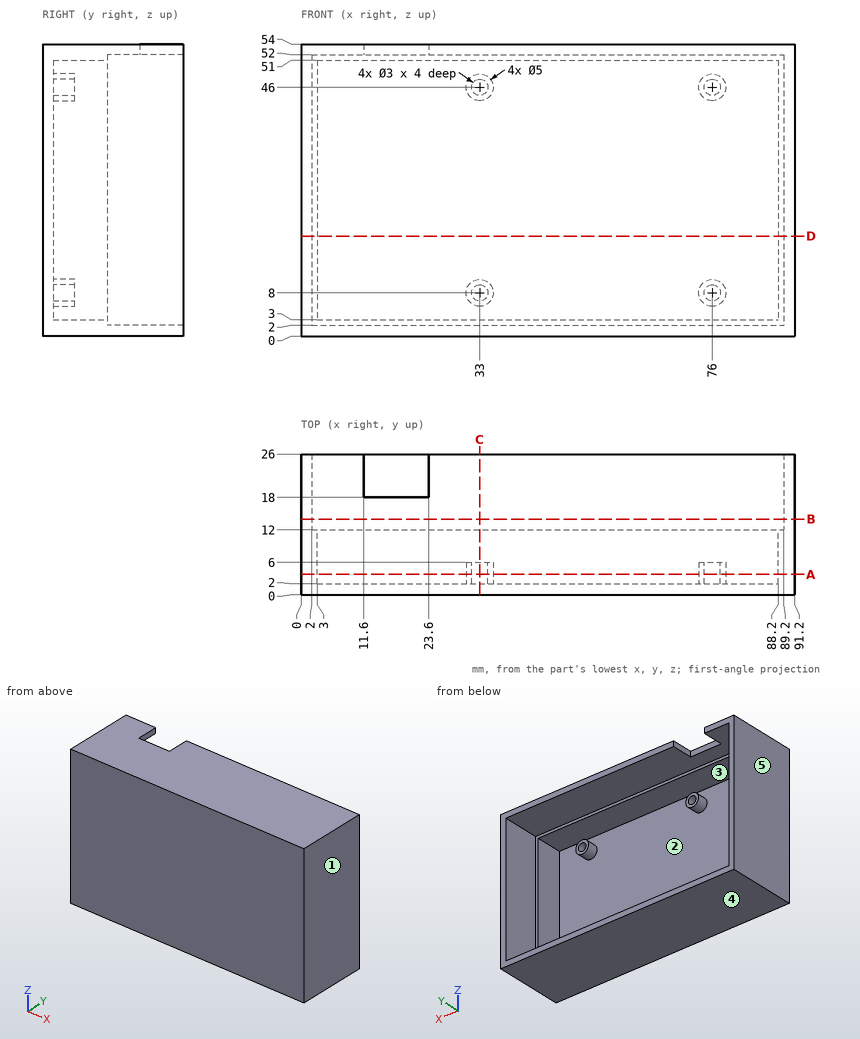
Study the drawing (mm; zero at the part's minimum x, y, z) and answer. A direction names the side the tool comes from. Give positions to 0.01 mm unless a question says otherwise; leave off trailing zeros. Write each loop counter-clockwise with the first axis right and the second up, starting at its lowest first coordinate (ties: lowest second). Pieces come first, ordered by that corner, then holes. Notation, with made-up numbers: (72.25, 60) - (101.25, 60) arc R15 cw to (101.25, 80) - close; hole circle Ø11 at (-27, -15). An arc over 180 degrees is marked (long way). Write item = value, one per line. Start each with the question number.
Item 1: Find section C-C (x = 33). Give the vertices of the cut face in (y, z), then the cut area to 3 significant figures.
Item 2: Find section A-A (y = 3.75). State how many separate pieces and enclosed holes the cut face has, then the cut area to 3 significant figures.
Item 3: Find the intervals of material crossed by probe 1 along X at (y, z) = (5.05, 8); probe 2 along Z at (x, y) = (76, 5.05); probe 3 along Z at (x, y) = (14.5, 2.75), in increasing order. Write a range as [from, to].
Item 4: Find section D-D (z = 18.5). Give the vertices of the cut face in (x, y), then the cut area to 3 significant figures.
Item 5: A tool of negligible diameter and unlimited length cuts with its end or side. For the marked faces 1 and 2, from which of +Z, -Z, +X, -X, +Y, -Y can it reach the whole face along a straight path? Write none if from no direction.
Item 6: Each of these flat-tipped pins is pushed along its axis until it touches: P1, Ø2, axis at x = 46, z = 29, coming from the +Y side; P2, Ø5.5, axis at x = 76, z = 45, coming from the +Y side; P3, Ø1.6, axis at x = 15, z = 53, coming from the +Y side. Where does it stop, or does it pass through?
Item 7: The mould has two halves that part along Z. Classify the marked faces 3, 4 and 5: +Z half, -Z half, draft (parallel to the pull), parting line (faces both ways), or undercut.
Item 8: Find section B-B (y = 14). Give the vertices of the cut face in (x, z), then the cut area to 3 significant figures.
Response:
q1.outline = (0, 0) - (26, 0) - (26, 2) - (12, 2) - (12, 3) - (2, 3) - (2, 5.5) - (6, 5.5) - (6, 6.5) - (2, 6.5) - (2, 9.5) - (6, 9.5) - (6, 10.5) - (2, 10.5) - (2, 43.5) - (6, 43.5) - (6, 44.5) - (2, 44.5) - (2, 47.5) - (6, 47.5) - (6, 48.5) - (2, 48.5) - (2, 51) - (12, 51) - (12, 52) - (26, 52) - (26, 54) - (0, 54) - close
q1.area = 240 mm²
q2.separate_pieces = 5
q2.enclosed_holes = 5
q2.area = 885 mm²
q3.probe_1 = [0, 3], [30.5, 31.5], [34.5, 35.5], [73.5, 74.5], [77.5, 78.5], [88.2, 91.2]
q3.probe_2 = [0, 3], [5.5, 6.5], [9.5, 10.5], [43.5, 44.5], [47.5, 48.5], [51, 54]
q3.probe_3 = [0, 3], [51, 54]
q4.outline = (0, 0) - (91.2, 0) - (91.2, 26) - (89.2, 26) - (89.2, 12) - (88.2, 12) - (88.2, 2) - (3, 2) - (3, 12) - (2, 12) - (2, 26) - (0, 26) - close
q4.area = 298 mm²
q5.face_1 = +Z, -Z, +X, +Y, -Y
q5.face_2 = +Y
q6.P1 = 2
q6.P2 = 6
q6.P3 = 18
q7.face_3 = undercut
q7.face_4 = -Z half
q7.face_5 = draft
q8.outline = (0, 0) - (91.2, 0) - (91.2, 54) - (0, 54) - close; hole (2, 2) - (89.2, 2) - (89.2, 52) - (2, 52) - close
q8.area = 565 mm²
